```python
from build123d import *

# Parameters (mm, degrees)
ESTRUSIONE_ESTRUSIONE1_DEPTH          = 3
FORO_SVASATO_PER_VITE_M4_1_AT_2_COUNT = 2
FORO_SVASATO_PER_VITE_M4_1_AT_2_PITCH = 95
FORO_SVASATO_PER_VITE_M3_1_AT_2_COUNT = 2
FORO_SVASATO_PER_VITE_M3_1_AT_2_PITCH = 60.5
FORO_SVASATO_PER_VITE_M3_1_AT_3_COUNT = 2
FORO_SVASATO_PER_VITE_M3_1_AT_3_PITCH = 88.782036471
FORO_SVASATO_PER_VITE_M3_1_AT_4_COUNT = 2
FORO_SVASATO_PER_VITE_M3_1_AT_4_PITCH = 38.5
M3_CLEARANCE_HOLE1_D                  = 3.6
M3_CLEARANCE_HOLE1_DEPTH              = 4
M3_CLEARANCE_HOLE1_TIP                = 1.081549114


with BuildPart() as part:
    # Schizzo1 → Estrusione-Estrusione1 (new body)
    with BuildSketch(Plane.XY):
        with BuildLine():
            Line((20.25, -47.5), (23.25, -47.5))
            Line((23.25, -47.5), (23.25, 47.5))
            Line((23.25, 47.5), (20.25, 47.5))
            ThreePointArc((20.25, 47.5), (0, 67.75), (-20.25, 47.5))
            Line((-20.25, 47.5), (-23.25, 47.5))
            Line((-23.25, 47.5), (-23.25, -47.5))
            Line((-23.25, -47.5), (-20.25, -47.5))
            ThreePointArc((-20.25, -47.5), (0, -67.75), (20.25, -47.5))
        make_face()
    extrude(amount=ESTRUSIONE_ESTRUSIONE1_DEPTH)

    # Schizzo5 → Foro svasato per Vite M4-1 (revolve, cut)
    with BuildSketch(Plane(origin=(0, 47.5, 0), x_dir=(0, 1, 0), z_dir=(1, 0, 0))):
        Polygon((0, 0), (0, 3), (2.25, 3), (2.25, 2.45), (4.7, 0), align=None)
    foro_svasato_per_vite_m4_1 = revolve(axis=Axis((0, 47.5, -6.35), (0, 0, 1)), mode=Mode.SUBTRACT)

    # Foro svasato per Vite M4-1 at 2: Foro svasato per Vite M4-1 ×2
    with Locations(*[(0, -i * FORO_SVASATO_PER_VITE_M4_1_AT_2_PITCH, 0) for i in range(1, FORO_SVASATO_PER_VITE_M4_1_AT_2_COUNT)]):
        add(foro_svasato_per_vite_m4_1, mode=Mode.SUBTRACT)

    # Schizzo8 → Foro svasato per Vite M3-1 (revolve, cut)
    with BuildSketch(Plane(origin=(19.25, 40, 0), x_dir=(0, 1, 0), z_dir=(1, 0, 0))):
        Polygon((0, 0), (0, 3), (1.7, 3), (1.7, 1.45), (3.15, 0), align=None)
    foro_svasato_per_vite_m3_1 = revolve(axis=Axis((19.25, 40, -6.35), (0, 0, 1)), mode=Mode.SUBTRACT)

    # Foro svasato per Vite M3-1 at 2: Foro svasato per Vite M3-1 ×2
    with Locations(*[(0, -i * FORO_SVASATO_PER_VITE_M3_1_AT_2_PITCH, 0) for i in range(1, FORO_SVASATO_PER_VITE_M3_1_AT_2_COUNT)]):
        add(foro_svasato_per_vite_m3_1, mode=Mode.SUBTRACT)

    # Foro svasato per Vite M3-1 at 3: Foro svasato per Vite M3-1 ×2
    with Locations(*[Vector(-0.43364628172754605, -0.9010831828104849, 0) * (i * FORO_SVASATO_PER_VITE_M3_1_AT_3_PITCH) for i in range(1, FORO_SVASATO_PER_VITE_M3_1_AT_3_COUNT)]):
        add(foro_svasato_per_vite_m3_1, mode=Mode.SUBTRACT)

    # Foro svasato per Vite M3-1 at 4: Foro svasato per Vite M3-1 ×2
    with Locations(*[(-i * FORO_SVASATO_PER_VITE_M3_1_AT_4_PITCH, 0, 0) for i in range(1, FORO_SVASATO_PER_VITE_M3_1_AT_4_COUNT)]):
        add(foro_svasato_per_vite_m3_1, mode=Mode.SUBTRACT)

    # M3 Clearance Hole1
    with Locations(Plane(origin=(0, 0, 0), x_dir=(-1, 0, 0), z_dir=(0, 0, -1))):
        with Locations((19.25, 0), (0, 65.25), (0, -65.25)):
            Hole(M3_CLEARANCE_HOLE1_D / 2, depth=M3_CLEARANCE_HOLE1_DEPTH)
            with Locations((0, 0, -(M3_CLEARANCE_HOLE1_DEPTH + M3_CLEARANCE_HOLE1_TIP / 2))):  # 118° drill point
                Cone(0, M3_CLEARANCE_HOLE1_D / 2, M3_CLEARANCE_HOLE1_TIP, mode=Mode.SUBTRACT)


solid = part.part
```
Could you check a few things on this model? Use its own coordinates, in mm. Coordinates: 2 decimals unless noted, no trailing zeros. Order: outer loops, then holes, each group sorted by start corner. A loop starts at its lowest first (then second) coordinate and runs counter-clockwise, first axis right, second up. Notation, with made-up numbers: M 89,-32.5 L 142,-32.5 A21 cw 142,1.5 Z; hole C 51.5,5 d11. An arc over 180 degrees is marked long. Use a Markdown table: item, result. Add a question column.
Q1. I want a section at A-A on y = 0. List the corners of the cut face in (x, z) for me.
Q2. I want a section at B-B on x = 6.5. List the corners of the cut face in (y, z) for me, then the cut area to 3 significant figures.
Q3. I want a section at D-D on x = -8. List the corners of the cut face in (y, z) for me, then the cut area to 3 significant figures.
Q4. If I drill on L1, parallel to X at y = -40, z = 2.6; L2, parallel to Y at x = 0, z = 2.9; L3, parallel to X at y = 41, z = 0.5, over which ranges is the centre line in solid material (lowest first)?
Q5. I want a section at C-C on y = -65.25. List the corners of the cut face in (x, z) for me.
Q6. We'd pull the mould along Y, two halves only. Please class faces 1 (the flat face through (22, 47.5, 1)), 2 (the cylindrical face through (19.2, 38.3, 2.2)), 3 (the flat face through (0, 1, 3)): pulls with the +Y half, pulls with the -Y half, needs draft (parallel to the pull), parting line crosses it, or undercut.
Q7. I'm going to push flat-ended pins straight in: pin 1 (1.5 mm diameter, centred on x = 18.5, z = 1.5, fed in from +Y); pin 2 (1 mm diameter, centred on x = 12.5, z = 1.5, fed in from -Y); pin 3 (3 mm diameter, centred on x = -19.25, y = -40, fed in from +Z); pin 4 (4.5 mm diameter, centred on x = 19.25, y = -20.5, fed in from -Z). Where does each tip first touch, or does it pass through?
Checked values:
| question | item | result |
|---|---|---|
| 1 | outline | M -23.25,0 L -21.05,0 L -21.05,3 L -23.25,3 Z; M -17.45,0 L 23.25,0 L 23.25,3 L -17.45,3 Z |
| 2 | outline | M -66.68,0 L 66.68,0 L 66.68,3 L -66.68,3 Z |
| 2 | area | 400 mm² |
| 3 | outline | M -66.1,0 L 66.1,0 L 66.1,3 L -66.1,3 Z |
| 3 | area | 397 mm² |
| 4 | L1 | -23.25 to -20.95, -17.55 to 23.25 |
| 4 | L2 | -67.75 to -67.05, -63.45 to -49.75, -45.25 to 45.25, 49.75 to 63.45, 67.05 to 67.75 |
| 4 | L3 | -23.25 to -21.7, -16.8 to 16.8, 21.7 to 23.25 |
| 5 | outline | M -9.75,0 L -1.8,0 L -1.8,3 L -9.75,3 Z; M 1.8,0 L 9.75,0 L 9.75,3 L 1.8,3 Z |
| 6 | face 1 | pulls with the +Y half |
| 6 | face 2 | undercut |
| 6 | face 3 | needs draft |
| 7 | pin 1 | y = 57.25 |
| 7 | pin 2 | y = -63.81 |
| 7 | pin 3 | through |
| 7 | pin 4 | z = 0.9 |
